from build123d import *

# Parameters (mm, degrees)
F2_W     = 11
F2_H     = 11
F3_DEPTH = 2
F4_SIZE  = 1.5


with BuildPart() as f1:
    # F0 (on Right) → F1 (revolve)
    with BuildSketch(Plane.YZ):
        Polygon((-1.675, 1), (-3.407051, 0), (0, 0), (0, 22.1), (-1.9, 22.1), (-1.9, 6.6), (-2, 5.6), (-2.5, 5.6), (-2.5, 4.6), (-1.675, 4.6), align=None)
    revolve(axis=Axis((0, 0, 11.05), (0, 0, -1)))

    # F2 (on Top) → F3 (join)
    with BuildSketch(Plane.XY):
        Rectangle(F2_W, F2_H)
    extrude(amount=-F3_DEPTH)

    # F4
    f4_edges = [f1.edges().sort_by_distance(p)[0] for p in [
        (-5.5, 5.5, -1),
        (5.5, 5.5, -1),
        (5.5, -5.5, -1),
        (-5.5, -5.5, -1),
    ]]
    chamfer(f4_edges, length=F4_SIZE)


solid = f1.part
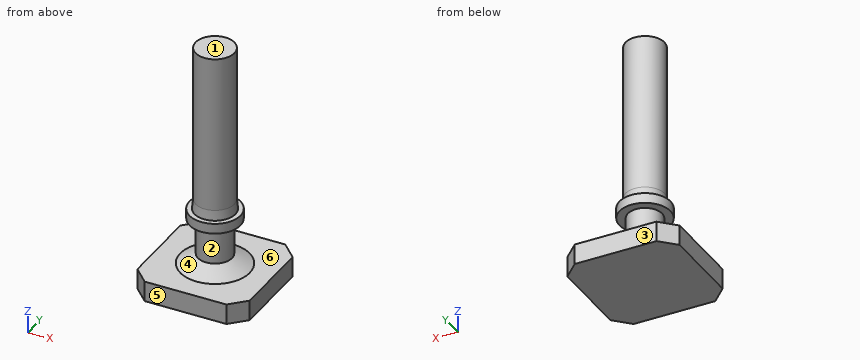
For this review, take the finished solid that the model builds, in its own axes (mm). Face numbers are marked on the shaded views. A direction names the side the tool comes from. Coordinates: 2 decimals unless noted, no trailing zeros. Loops run counter-clockwise (first coordinate to the right, second up) from the corner with the lowest first, then second, coordinate; pieces in that order, holes last. Notation, with made-up numbers: (-29, 74) - (-18, 74) arc R7 ccw to (-18, 87) - close; hole circle Ø5 at (3.5, 39). An arc over 180 degrees is marked (long way). Use a Markdown table: item, result. Add a question column.
Item 1: We need section C-C (z = 20.25). Give the boundary of the cut face in (x, y), and give its area (3 significant figures).
Item 2: For line 1 (Z direction, x = 2, y = 4); line 2 (X direction, y = -1.5, z = 15.5); line 3 (Y direction, x = -1.25, z = 17.5), list the stretches that pass through material, from the lowest coordinate up.
Item 3: We need section D-D (y = 5.25). Give the boundary of the cut face in (x, z), and give its area (3 significant figures).
Item 4: We need section A-A (x = 0). Give the boundary of the cut face in (y, z) (3 decimals).
Item 5: Insertion check: pin 1 Ø1 at (x, y) = (2.5, 1.5) entering from +Z; pin 2 Ø5.5 at (x, y) = (2.5, -2.5) entering from +Z; pin 3 Ø5 at (x, z) = (-2, 11.5) entering from +Y; pin 4 Ø5 at (x, z) = (0.5, 19.5) entering from -Y. Each pin has a flat end and moves straight along its axis. Give the tip position at first contact, or say it passes through.
Item 6: Mouldability with a two-part tool opening along Z and no side actions: class the marked faces 1, 2 and 3 as pulls with the +Z half, pulls with the -Z half, needs draft (parallel to the pull), parting line crosses it, or undercut.
Item 7: Tool access review of the marked faces 4, 5 and 6: name each direction out of +Z, -Z, +X, -X, +Y, -Y from which nothing blocks a thin tool from reaching the whole face with its end or side.
Results list:
| question | item | result |
|---|---|---|
| 1 | outline | circle Ø3.8 at (0, 0) |
| 1 | area | 11.3 mm^2 |
| 2 | line 1 | z = -2 to 0 |
| 2 | line 2 | x = -1.17 to 1.17 |
| 2 | line 3 | y = -1.43 to 1.43 |
| 3 | outline | (-4.25, -2) - (4.25, -2) - (4.25, 0) - (-4.25, 0) - close |
| 3 | area | 17.0 mm^2 |
| 4 | outline | (-5.5, -2) - (5.5, -2) - (5.5, 0) - (3.407, 0) - (1.675, 1) - (1.675, 4.6) - (2.5, 4.6) - (2.5, 5.6) - (2, 5.6) - (1.9, 6.6) - (1.9, 22.1) - (-1.9, 22.1) - (-1.9, 6.6) - (-2, 5.6) - (-2.5, 5.6) - (-2.5, 4.6) - (-1.675, 4.6) - (-1.675, 1) - (-3.407, 0) - (-5.5, 0) - close |
| 5 | pin 1 | stops at z = 5.6 |
| 5 | pin 2 | stops at z = 22.1 |
| 5 | pin 3 | stops at y = 1.9 |
| 5 | pin 4 | stops at y = -1.9 |
| 6 | face 1 | pulls with the +Z half |
| 6 | face 2 | undercut |
| 6 | face 3 | needs draft |
| 7 | face 4 | none |
| 7 | face 5 | +Z, -Z, +X, -X, -Y |
| 7 | face 6 | +Z |
